Read the model definition and answer for the solid it produces. Units are mm, in the model's axes. A direction names the side the tool comes from. Coordinates: 2 decimals unless noted, no trailing zeros. Loops run counter-clockwise (first coordinate to the right, second up) from the corner with the lowest first, then second, coordinate; pieces in that order, holes last. Notation, with made-up numbers: (-5, -5) -> (13, -5) arc R24 cw to (13, 9) -> close; hole circle Ø7 at (58.5, 28.5). An arc over 180 degrees is marked (long way). Answer as a JSON object with one key per item and string values. Group by question number.
1) Flat-ended cylindrical pins translate along their axes: P1, Ø2, axis at x = 15.5, y = -35.5, coming from the +Z side; P2, Ø4, axis at x = 9, z = 32, coming from the +Y side. Find the tip coordinate at first contact, or state that the pin passes through.
2) Determine the mould class of faces 1 (the face through (3, -32, 30)), 2 (the face through (14, -38, 30)), 3 (the face through (3, 0, 30)) for opening direction Y: released by +Y, released by -Y, zero draft, split by the parting line, or undercut.
3) Consider probe 1 along Y at (x, z) = (5.75, 13); probe 2 along Y at (x, z) = (10, 34); probe 3 along X at (y, z) = (-34, 32). Determine where each line is inside the solid, lowest interval first. Write a range as [from, to].
4) Section B-B, the plane x = 10 is taken. Give the vertices of the cut face in (y, z).
5) Which of the six approach directions +Z, -Z, +X, -X, +Y, -Y give full straight-line access (tool end or side, diameter ignored) to faces 4 (the face through (10, -24, 60)), 5 (the face through (3, -7, 30)), 6 (the face through (14, -27, 30))?
6) Section A-A, the plane y = -20 is taken. Give the vertices of the cut face in (x, z).
from build123d import *

# Parameters (mm, degrees)
SKETCH_2_R      = 3.4
EXTRUDE_1_DEPTH = 60


with BuildPart() as part:
    # 草图2 → 凸台-拉伸1 (new body)
    with BuildSketch(Plane.XY):
        Polygon((0, 0), (6, 0), (6, -4), (3, -4), (3, -11), (6, -11), (6, -15), (14, -15), (14, -11), (17, -11), (17, -4), (14, -4), (14, 0), (20, 0), (20, -40), (14, -40), (14, -36), (17, -36), (17, -29), (14, -29), (14, -25), (6, -25), (6, -29), (3, -29), (3, -36), (6, -36), (6, -40), (0, -40), align=None)
        with Locations(Location((10, -20, 0), (0, 0, 180))):
            Circle(SKETCH_2_R, mode=Mode.SUBTRACT)
    extrude(amount=EXTRUDE_1_DEPTH)


solid = part.part
Determined:
{
 "1": {"P1": "z = 60", "P2": "y = -15"},
 "2": {"face 1": "undercut", "face 2": "zero draft", "face 3": "released by +Y"},
 "3": {"probe 1": "[-40, -36], [-29, -11], [-4, 0]", "probe 2": "[-25, -23.4], [-16.6, -15]", "probe 3": "[0, 3], [17, 20]"},
 "4": {"outline": "(-25, 0) -> (-23.4, 0) -> (-23.4, 60) -> (-25, 60) -> close; (-16.6, 0) -> (-15, 0) -> (-15, 60) -> (-16.6, 60) -> close"},
 "5": {"face 4": "+Z, +X, -X, +Y, -Y", "face 5": "+Z, -Z", "face 6": "+Z, -Z, -Y"},
 "6": {"outline": "(0, 0) -> (6.6, 0) -> (6.6, 60) -> (0, 60) -> close; (13.4, 0) -> (20, 0) -> (20, 60) -> (13.4, 60) -> close"}
}
